```python
from build123d import *

# Parameters (mm, degrees)
F1_DEPTH         = 3.175
F3_DEPTH         = 25.4
F4_W             = 97.3040463274
F4_H             = 1.905
F5_DEPTH         = 12.7
F6_W             = 40.64
F6_H             = 25.4
F7_DEPTH         = 11.43
F8_W             = 31.75
F8_H             = 17.78
F9_DEPTH         = 3.175
F10_W            = 31.75
F10_H            = 4.445
F11_DEPTH        = 27.305
F12_W            = 31.75
F12_H            = 1.27
F13_DEPTH        = 2.54
F15_DEPTH        = 31.75
F15_COPIES_COUNT = 3
F15_COPIES_PITCH = 0.5207
F17_DEPTH        = 38.1
F18_DEPTH        = 6.35
F19_R            = 5.08


# Not quite as in the source:
# - a pattern or mirror of a feature is missing from the dataset's text; its kind, count and spacing are read off the source's solid


with BuildPart() as f1:
    # F0 (on Top) → F1 (new body)
    with BuildSketch(Plane.XY):
        Polygon((3.175, 48.1711), (-3.175, 48.1711), (-51.3461, 0), (-48.6520231637, -2.6940768363), (48.6520231637, -2.6940768363), (51.3461, 0), align=None)
    extrude(amount=F1_DEPTH)

    # F2 (on face) → F3 (join)
    with BuildSketch(Plane.XY.offset(3.175)):
        Polygon((-3.175, 48.1711), (-51.3461, 0), (-50.8970871939, -0.4490128061), (-2.916877582, 47.5311968059), (2.916871896, 47.5312024919), (50.8970871939, -0.4490128061), (51.3461, 0), (3.175, 48.1711), align=None)
    extrude(amount=F3_DEPTH)

    # F4 (on face) → F5 (join)
    with BuildSketch(Plane(origin=(0, 0, 0), x_dir=(1, 0, 0), z_dir=(0, 0, -1))):
        with Locations((0, 1.7415768363)):
            Rectangle(F4_W, F4_H)
    extrude(amount=F5_DEPTH)

    # F6 (on face) → F7 (join)
    with BuildSketch(Plane(origin=(0, 0, 0), x_dir=(1, 0, 0), z_dir=(0, 0, -1))):
        with Locations((-0.0357092768, -11.9109231637)):
            Rectangle(F6_W, F6_H)
    extrude(amount=F7_DEPTH)

    # F8 (on face) → F9 (cut, through all)
    with BuildSketch(Plane(origin=(0, 0, 0), x_dir=(1, 0, 0), z_dir=(0, 0, -1))):
        with Locations((-0.0357092768, -10.0059231637)):
            Rectangle(F8_W, F8_H)
    extrude(amount=-F9_DEPTH, mode=Mode.SUBTRACT)

    # F10 (on face) → F11 (cut, through all)
    with BuildSketch(Plane(origin=(0, 24.6109231637, 0), x_dir=(-1, 0, 0), z_dir=(0, 1, 0))):
        with Locations((-7.74733e-05, -2.2225)):
            Rectangle(F10_W, F10_H)
    extrude(amount=-F11_DEPTH, mode=Mode.SUBTRACT)

    # F12 (on face) → F13 (join)
    with BuildSketch(Plane.XZ.offset(2.6940768363)):
        with Locations((7.74733e-05, 0.635)):
            Rectangle(F12_W, F12_H)
    extrude(amount=F13_DEPTH)

    # F14 (on face) → F15 (join, through all)
    with BuildSketch(Plane.YZ.offset(15.8750774733)):
        Polygon((-3.6032828125, -0.3642210371), (-3.0831212644, 0), (-3.6032828125, 0), align=None)
    f15 = extrude(amount=-F15_DEPTH)

    # F15_copies: F15 ×3
    with Locations(*[(0, -i * F15_COPIES_PITCH, 0) for i in range(1, F15_COPIES_COUNT)]):
        add(f15)

    # F16 (on face) → F17 (join)
    with BuildSketch(Plane.YZ.offset(15.8750774733)):
        with BuildLine():
            Line((-9.1575253509, 2.9035897025), (-10.161578661, 2.1184348754))
            ThreePointArc((-10.161578661, 2.1184348754), (-7.9158691733, 0.5520507884), (-5.2340768363, 0))
            Line((-5.2340768363, 0), (-5.2340768363, 1.27))
            ThreePointArc((-5.2340768363, 1.27), (-7.3590511634, 1.6947115498), (-9.1575253509, 2.9035897025))
        make_face()
    extrude(amount=-F17_DEPTH)

    # F16 (on face) → F18 (join)
    with BuildSketch(Plane.YZ.offset(15.8750774733)):
        with BuildLine():
            Line((-9.1575253509, 2.9035897025), (-10.161578661, 2.1184348754))
            ThreePointArc((-10.161578661, 2.1184348754), (-7.9158691733, 0.5520507884), (-5.2340768363, 0))
            Line((-5.2340768363, 0), (-5.2340768363, 1.27))
            ThreePointArc((-5.2340768363, 1.27), (-7.3590511634, 1.6947115498), (-9.1575253509, 2.9035897025))
        make_face()
    extrude(amount=F18_DEPTH)

    # F19
    f19_edges = [f1.edges().sort_by_distance(p)[0] for p in [
        (-48.652023, -1.741577, -12.7),
        (48.652023, -1.741577, -12.7),
    ]]
    fillet(f19_edges, radius=F19_R)


solid = f1.part
```
Design review of the part built by this model. Coordinates are the model's own, in mm. A direction names the side the tool comes from. Round coordinates to 2 decimals unless told otherwise and drop trailing zeros. Order: outer loops, then holes, each group sorted by start corner. A loop starts at its lowest first (then second) coordinate and runs counter-clockwise, first axis right, second up. Notation, with made-up numbers: (13.25, 64.25) - (61.25, 64.25) arc R16 cw to (61.25, 86.25) - close; hole circle Ø7 at (-10, 68.5). An arc over 180 degrees is marked (long way). Return JSON: item names as keys, results as strings.
Q1. Consider section B-B on x = -8.5. Give the number of separate pieces and of enclosed holes in the cut face, plus the area to 3 significant figures.
Computed values:
{"separate pieces": "3", "enclosed holes": "0", "area": "314 mm2"}
Q2. Wall thickness on L1, parallel to X at y = 5.5, z = -2; L2, parallel to Z at x = -5, y = 21 (3 decimals); L3, parallel to Y at x = 22.5, z = -7.5: over which ranges is each line inside the solid? List them lowest first. Write a range as [from, to].
Computed values:
{"L1": "x = [-20.36, -15.87], [15.88, 20.28]", "L2": "z = [-11.43, -4.445], [0, 3.175]", "L3": "y = [-2.69, -0.79]"}
Q3. Machinability: for faces 1 (the flat face through (0, 11, -4.445)), 2 (the flat face through (22.225, -8, 1)), 3 (the flat face through (15.839, 10, 2)), which of the approach directions +Z, -Z, +X, -X, +Y, -Y give a long, thin tool a straight path to every point of the face, cutting with its end or side? Answer none if there is none.
Computed values:
{"face 1": "+Y, -Y", "face 2": "+Z, -Z, +X, -Y", "face 3": "+Z"}
Q4. Consider section C-C on z = 22.5. Write out the cut boundary in (x, y) (3 decimals), plus the area to 3 significant figures.
Computed values:
{"outline": "(-51.346, 0) - (-50.897, -0.449) - (-2.917, 47.531) - (2.917, 47.531) - (50.897, -0.449) - (51.346, 0) - (3.175, 48.171) - (-3.175, 48.171) - close", "area": "90.2 mm2"}
Q5. Consider section D-D on y = 9.5. Write out the cut boundary in (x, z) (3 decimals), plus the area to 3 significant figures.
Computed values:
{"outline": "(-41.846, 0) - (-20.356, 0) - (-20.356, -11.43) - (20.284, -11.43) - (20.284, 0) - (41.846, 0) - (41.846, 28.575) - (40.948, 28.575) - (40.948, 3.175) - (15.839, 3.175) - (15.839, 0) - (15.875, 0) - (15.875, -4.445) - (-15.875, -4.445) - (-15.875, 0) - (-15.911, 0) - (-15.911, 3.175) - (-40.948, 3.175) - (-40.948, 28.575) - (-41.846, 28.575) - close", "area": "534 mm2"}
Q6. Consider section A-A on z = -2. Write out the cut boundary in (x, y).
Computed values:
{"outline": "(-48.65, -2.69) - (-15.87, -2.69) - (-15.87, 24.61) - (-20.36, 24.61) - (-20.36, -0.79) - (-48.65, -0.79) - close; (15.88, -2.69) - (48.65, -2.69) - (48.65, -0.79) - (20.28, -0.79) - (20.28, 24.61) - (15.88, 24.61) - close"}
Q7. The part is to be moulded in two halves that separate along X. For faces 4 (the flat face through (0, 48.171, 14)), 5 (the flat face through (15.875, 11, -2)), 6 (the flat face through (27.598, 23.748, 14.087)), say which applies: pulls with the +X half, pulls with the -X half, needs draft (parallel to the pull), parting line crosses it, or undercut.
Computed values:
{"face 4": "needs draft", "face 5": "undercut", "face 6": "pulls with the +X half"}
Q8. For pin 1 Ø12.5 at (x, z) = (24, -2.5) entering from -Y; pin 2 Ø5 at (x, z) = (20, 15) entering from +Y; pin 3 Ø12 at (x, z) = (-35, 0) entering from +Y; pin 4 Ø22 at (x, y) = (5, 5.5) entering from +Z (3 decimals), all flat-tipped, find the tip position at first contact; note any pin that passes through.
Computed values:
{"pin 1": "stops at y = -10.16", "pin 2": "stops at y = 33.85", "pin 3": "stops at y = 22.35", "pin 4": "stops at z = 3.175"}
